from build123d import *

# Parameters (mm, degrees)
ESQUISSE1_W                                   = 30
ESQUISSE1_H                                   = 26
ESQUISSE1_R                                   = 10
BOSS_EXTRU_1_DEPTH                            = 6
ESQUISSE2_R                                   = 10.5
ENL_V_MAT_EXTRU_1_DEPTH                       = 5
TROU_POUR_TARAUDAGE_POUR_TROU_TARAUD_M2_D     = 1.6
TROU_POUR_TARAUDAGE_POUR_TROU_TARAUD_M2_DEPTH = 10
TROU_POUR_TARAUDAGE_POUR_TROU_TARAUD_M2_TIP   = 0.480688495
TROU_POUR_TARAUDAGE_POUR_TROU_TARAUD_2_D      = 1.6
TROU_POUR_TARAUDAGE_POUR_TROU_TARAUD_2_DEPTH  = 10
TROU_POUR_TARAUDAGE_POUR_TROU_TARAUD_2_TIP    = 0.480688495


with BuildPart() as part:
    # Esquisse1 → Boss.-Extru.1 (new body)
    with BuildSketch(Plane.XY):
        with Locations((15, 13)):
            Rectangle(ESQUISSE1_W, ESQUISSE1_H)
        with Locations((15, 13)):
            Circle(ESQUISSE1_R, mode=Mode.SUBTRACT)
    extrude(amount=BOSS_EXTRU_1_DEPTH)

    # Esquisse2 → Enlèv. mat.-Extru.1 (cut)
    with BuildSketch(Plane.XY.offset(6)):
        with Locations((15, 13)):
            Circle(ESQUISSE2_R)
    extrude(amount=-ENL_V_MAT_EXTRU_1_DEPTH, mode=Mode.SUBTRACT)

    # Trou pour taraudage pour trou taraud_ M2
    with Locations(Plane(origin=(0, 26, 0), x_dir=(1, 0, 0), z_dir=(0, 1, 0))):
        with Locations((4, -3), (26, -3)):
            Hole(TROU_POUR_TARAUDAGE_POUR_TROU_TARAUD_M2_D / 2, depth=TROU_POUR_TARAUDAGE_POUR_TROU_TARAUD_M2_DEPTH)
            with Locations((0, 0, -(TROU_POUR_TARAUDAGE_POUR_TROU_TARAUD_M2_DEPTH + TROU_POUR_TARAUDAGE_POUR_TROU_TARAUD_M2_TIP / 2))):  # 118° drill point
                Cone(0, TROU_POUR_TARAUDAGE_POUR_TROU_TARAUD_M2_D / 2, TROU_POUR_TARAUDAGE_POUR_TROU_TARAUD_M2_TIP, mode=Mode.SUBTRACT)

    # Trou pour taraudage pour trou taraud 2
    with Locations(Plane(origin=(0, 0, 0), x_dir=(-1, 0, 0), z_dir=(0, -1, 0))):
        with Locations((-26, -3), (-4, -3)):
            Hole(TROU_POUR_TARAUDAGE_POUR_TROU_TARAUD_2_D / 2, depth=TROU_POUR_TARAUDAGE_POUR_TROU_TARAUD_2_DEPTH)
            with Locations((0, 0, -(TROU_POUR_TARAUDAGE_POUR_TROU_TARAUD_2_DEPTH + TROU_POUR_TARAUDAGE_POUR_TROU_TARAUD_2_TIP / 2))):  # 118° drill point
                Cone(0, TROU_POUR_TARAUDAGE_POUR_TROU_TARAUD_2_D / 2, TROU_POUR_TARAUDAGE_POUR_TROU_TARAUD_2_TIP, mode=Mode.SUBTRACT)


solid = part.part
The model under review builds one solid part; all positions refer to its coordinate system, in mm. A direction names the side the tool comes from. Round coordinates to 2 decimals unless told otherwise and drop trailing zeros. Order: outer loops, then holes, each group sorted by start corner. A loop starts at its lowest first (then second) coordinate and runs counter-clockwise, first axis right, second up. Notation, with made-up numbers: (-12.5, 57.25) -> (9.5, 57.25) arc R16 ccw to (9.5, 84.25) -> close; hole circle Ø1 at (50.25, 45.25). An arc over 180 degrees is marked (long way). Use CSV: the item, a comma, the result in double quotes. Start each with the question number.
(1) Wall thickness on probe 1 along Z at (x, y) = (4, 4.5); probe 2 along Y at (x, z) = (15, 3.45); probe 3 along X at (y, z) = (5.25, 3): over which ranges is each line inside the solid? List them lowest first. Write a range as from..to.
(2) Consider section B-B on x = 15. Write out the cut boundary in (y, z), and give its area (3 significant figures).
(3) Tool access review of faces 5 (the face through (3.37, 5.07, 3.49)), 6 (the face through (20, 4, 1)), 7 (the face through (4.8, 13.2, 0)), 8 (the face through (25.237, 20.93, 2.76)): name each direction out of +Z, -Z, +X, -X, +Y, -Y from which nothing blocks a thin tool from reaching the whole face with its end or side.
(4) Mouldability with a two-part tool opening along X and no side actions: class faces 1 (the face through (0, 13, 3)), 2 (the face through (4.8, 16.1, 6)), 3 (the face through (26.763, 5.07, 2.76)), 4 (the face through (24.54, 16, 0.49)) as pulls with the +X half, pulls with the -X half, needs draft (parallel to the pull), parting line crosses it, or undercut.
(5) Consider section A-A on y = 21.75. Write out the cut boundary in (x, z), and give its area (3 significant figures).
(6) Consider section C-C on y = 13. Write out the cut boundary in (x, z).
(7) Insertion check: pin 1 (1 mm diameter, centred on x = 26, z = 3, fed in from +Y); pin 2 (1.4 mm diameter, centred on x = 4, z = 3, fed in from +Y); pin 3 (5 mm diameter, centred on x = 13, y = 19.5, fed in from +Z). Each pin has a flat end and moves straight along its axis. Give the tip position at first contact, or say it passes through.
(8) Consider section D-D on y = 8.5. Write out the cut boundary in (x, z).
Responses:
1,probe 1,"0..2.2, 3.8..6"
1,probe 2,"0..2.5, 23.5..26"
1,probe 3,"0..3.2, 4.8..7.92, 22.08..25.2, 26.8..30"
2,outline,"(0, 0) -> (3, 0) -> (3, 1) -> (2.5, 1) -> (2.5, 6) -> (0, 6) -> close; (23, 0) -> (26, 0) -> (26, 6) -> (23.5, 6) -> (23.5, 1) -> (23, 1) -> close"
2,area,"31.0 mm²"
3,face 5,"-Y"
3,face 6,"+Z"
3,face 7,"-Z, +X, -X, +Y, -Y"
3,face 8,"+Y"
4,face 1,"pulls with the -X half"
4,face 2,"needs draft"
4,face 3,"undercut"
4,face 4,"undercut"
5,outline,"(0, 0) -> (10.16, 0) -> (10.16, 1) -> (9.2, 1) -> (9.2, 6) -> (0, 6) -> close; (19.84, 0) -> (30, 0) -> (30, 6) -> (20.8, 6) -> (20.8, 1) -> (19.84, 1) -> close; hole circle Ø1.6 at (4, 3); hole circle Ø1.6 at (26, 3)"
5,area,"108 mm²"
6,outline,"(0, 0) -> (5, 0) -> (5, 1) -> (4.5, 1) -> (4.5, 6) -> (0, 6) -> close; (25, 0) -> (30, 0) -> (30, 6) -> (25.5, 6) -> (25.5, 1) -> (25, 1) -> close"
7,pin 1,"y = 15.82"
7,pin 2,"y = 15.94"
7,pin 3,"through"
8,outline,"(0, 0) -> (6.07, 0) -> (6.07, 1) -> (5.51, 1) -> (5.51, 6) -> (0, 6) -> close; (23.93, 0) -> (30, 0) -> (30, 6) -> (24.49, 6) -> (24.49, 1) -> (23.93, 1) -> close; hole circle Ø1.6 at (4, 3); hole circle Ø1.6 at (26, 3)"
